from build123d import *

# Parameters (mm, degrees)
F0_W      = 110.1217
F0_H      = 132.1181
F1_DEPTH  = 39.9542
F2_W      = 132.1181
F2_H      = 38.6842
F3_DEPTH  = 18.9992
F4_W      = 132.1181
F4_H      = 38.6842
F5_DEPTH  = 18.9992
F6_W      = 18.9992
F6_H      = 132.1181
F7_DEPTH  = 1.271
F8_W      = 18.9992
F8_H      = 132.1181
F9_DEPTH  = 1.271
F10_W     = 67.0433
F10_H     = 127.0381
F11_DEPTH = 37.4142


with BuildPart() as f1:
    # F0 (on Top) → F1 (new body)
    with BuildSketch(Plane.XY):
        Rectangle(F0_W, F0_H)
    extrude(amount=F1_DEPTH)

    # F2 (on face) → F3 (cut)
    with BuildSketch(Plane(origin=(-55.06085, 0, 0), x_dir=(0, -1, 0), z_dir=(-1, 0, 0))):
        with Locations((0, 19.3421)):
            Rectangle(F2_W, F2_H)
    extrude(amount=-F3_DEPTH, mode=Mode.SUBTRACT)

    # F4 (on face) → F5 (cut)
    with BuildSketch(Plane.YZ.offset(55.06085)):
        with Locations((0, 19.3421)):
            Rectangle(F4_W, F4_H)
    extrude(amount=-F5_DEPTH, mode=Mode.SUBTRACT)

    # F6 (on face) → F7 (cut, through all)
    with BuildSketch(Plane(origin=(0, 0, 38.6842), x_dir=(1, 0, 0), z_dir=(0, 0, -1))):
        with Locations((-45.56125, 0)):
            Rectangle(F6_W, F6_H)
    extrude(amount=-F7_DEPTH, mode=Mode.SUBTRACT)

    # F8 (on face) → F9 (cut, through all)
    with BuildSketch(Plane(origin=(0, 0, 38.6842), x_dir=(1, 0, 0), z_dir=(0, 0, -1))):
        with Locations((45.56125, 0)):
            Rectangle(F8_W, F8_H)
    extrude(amount=-F9_DEPTH, mode=Mode.SUBTRACT)

    # F10 (on face) → F11 (cut)
    with BuildSketch(Plane.XY.offset(39.9542)):
        Rectangle(F10_W, F10_H)
    extrude(amount=-F11_DEPTH, mode=Mode.SUBTRACT)


solid = f1.part
Check sheet for the modelled part. Datum: model origin and axes. Units: mm. A direction names the side the tool comes from. Coordinates: 2 decimals unless noted, no trailing zeros. Write each loop counter-clockwise with the first axis right and the second up, starting at its lowest first coordinate (ties: lowest second). Pieces come first, ordered by that corner, then holes.
Item 1: Cross-section at A-A on y = -12. Record the boundary of the cut face in (x, z), then the cut area to 3 significant figures.
Numbers:
outline: (-36.06, 0) - (36.06, 0) - (36.06, 39.95) - (33.52, 39.95) - (33.52, 2.54) - (-33.52, 2.54) - (-33.52, 39.95) - (-36.06, 39.95) - close
area: 373 mm2
Item 2: Cross-section at B-B on z = 30.5. Record the boundary of the cut face in (x, y).
Numbers:
outline: (-36.06, -66.06) - (36.06, -66.06) - (36.06, 66.06) - (-36.06, 66.06) - close; hole (-33.52, -63.52) - (33.52, -63.52) - (33.52, 63.52) - (-33.52, 63.52) - close
Item 3: Access from +Z, -Z, +X, -X, +Y, -Y to the whole of each face (thin tool, end or side, straight path). Record for faces 4 (the face through (-1, -66.059, 20)), 5 (the face through (0, 1, 2.54)).
Numbers:
face 4: +Z, -Z, +X, -X, -Y
face 5: +Z
Item 4: Scan lines: probe 1 along X at (y, z) = (29.5, 12); probe 2 along Y at (x, z) = (-25.5, 19); probe 3 along Z at (x, y) = (-10, -47.5). Record each from-to range of solid material in increasing order.
Numbers:
probe 1: x = -36.06 to -33.52, 33.52 to 36.06
probe 2: y = -66.06 to -63.52, 63.52 to 66.06
probe 3: z = 0 to 2.54
Item 5: Depth check by flat-ended pin: pin 1 Ø12 at (x, y) = (10.5, 47.5) entering from +Z. Enter the tip coordinate at first touch or a pass-through.
Numbers:
pin 1: stops at z = 2.54
Item 6: Cross-section at C-C on x = -17. Record the boundary of the cut face in (y, z).
Numbers:
outline: (-66.06, 0) - (66.06, 0) - (66.06, 39.95) - (63.52, 39.95) - (63.52, 2.54) - (-63.52, 2.54) - (-63.52, 39.95) - (-66.06, 39.95) - close
Item 7: Mould release check, pull along Y, two halves, no side actions. Record for faces 1 (the face through (-1, 66.059, 20)), 2 (the face through (0, -63.519, 22)), 3 (the face through (-36.062, 1, 20)): released by +Y, released by -Y, zero draft, split by the parting line, or undercut.
Numbers:
face 1: released by +Y
face 2: undercut
face 3: zero draft
